Answer from the drawing. Dimensions are ordinates in mm from the lowest x, y and z of the part. Coordinates: 2 decimals unless noted, no trailing zeros. Write each loop counter-clockwise with the first axis right and the second up, starting at its lowest first coordinate (ties: lowest second). Pieces come first, ordered by that corner, then holes. Notation, with made-up numbers: (-4.75, -12) - (41.25, -12) arc R12 ccw to (41.25, 1) - close; hole circle Ø8 at (64, 31). An arc over 180 degrees is marked (long way). Return JSON: item names as keys, results as strings.
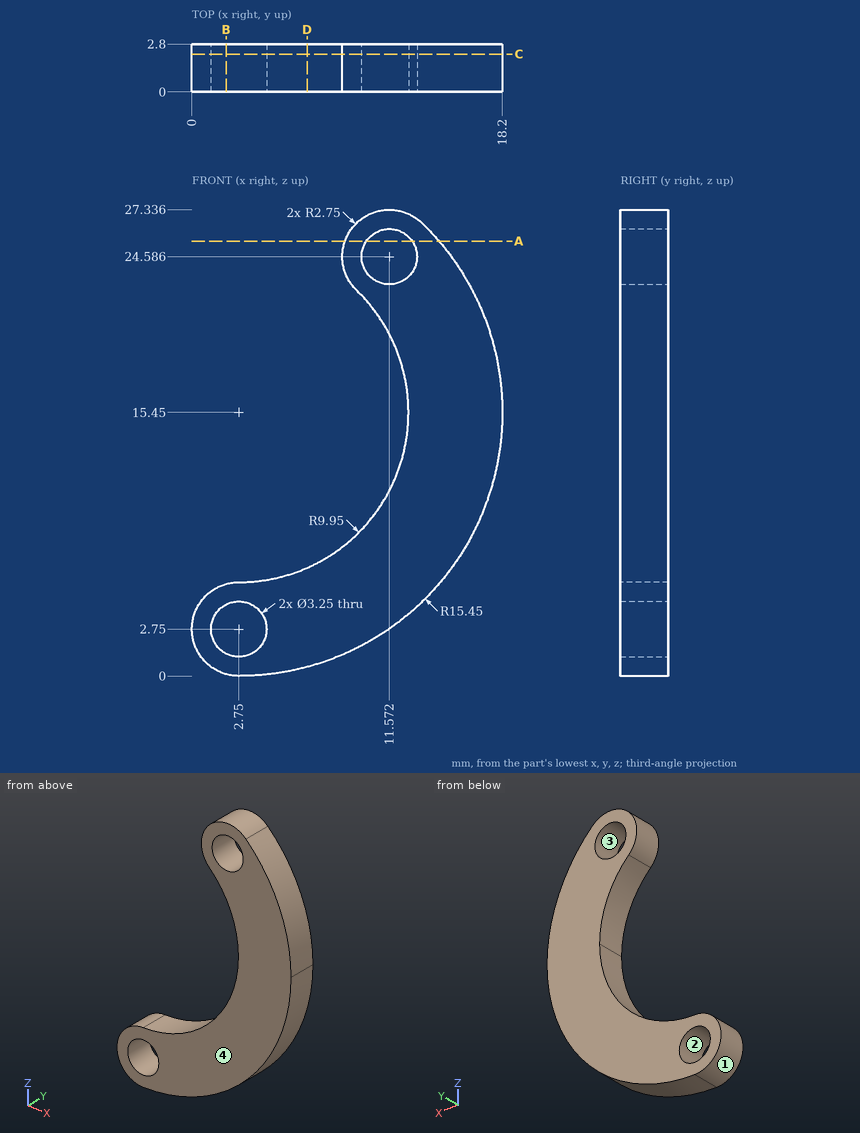
(1) A cutting plane is placed at B-B (x = 2). Determine the outline of the cut face in (y, z) (1 decimal).
Answer:
{"outline": "(0, 0.1) - (2.8, 0.1) - (2.8, 1.3) - (0, 1.3) - close; (0, 4.2) - (2.8, 4.2) - (2.8, 5.4) - (0, 5.4) - close"}
(2) Straight lines are drawn through the part: line 1 (Z direction, x = 2.75, y = 0.6) (1 decimal); line 2 (Z direction, x = 11, y = 1.2) (1 decimal); line 3 (Z direction, x = 4, y = 0.65). For each, find the intervals that lie inside material, in ascending order. Write a range as from..to.
Answer:
{"line 1": "0..1.1, 4.4..5.5", "line 2": "2.4..9.9, 21..23.1, 26.1..27.3", "line 3": "0.05..1.71, 3.79..5.58"}
(3) A cutting plane is placed at A-A (z = 25.5). Determine the outline of the cut face in (x, y) (1 decimal).
Answer:
{"outline": "(9, 0) - (10.2, 0) - (10.2, 2.8) - (9, 2.8) - close; (12.9, 0) - (14.5, 0) - (14.5, 2.8) - (12.9, 2.8) - close"}
(4) A cutting plane is placed at C-C (y = 2.2). State how many separate pieces and enclosed holes the cut face has, and give its area (3 significant figures).
Answer:
{"separate pieces": "1", "enclosed holes": "2", "area": "173 mm²"}
(5) A cutting plane is placed at D-D (x = 6.75). Determine the outline of the cut face in (y, z), and give its area (3 significant figures).
Answer:
{"outline": "(0, 0.53) - (2.8, 0.53) - (2.8, 6.34) - (0, 6.34) - close", "area": "16.3 mm²"}
(6) Determine the mould class of the marked faces 1, 2, 3 and 4 for opening direction Z: +Z half, -Z half, draft (parallel to the pull), parting line (faces both ways), or undercut.
Answer:
{"face 1": "parting line", "face 2": "undercut", "face 3": "undercut", "face 4": "draft"}
(7) Flat-ended cylindrical pins translate along their axes: P1, Ø3, axis at x = 2.75, z = 2.75, coming from the -Y side; P2, Ø1, axis at y = 2, z = 17, coming from the -X side. Find the tip coordinate at first contact, or state that the pin passes through.
Answer:
{"P1": "through", "P2": "x = 12.49"}
